The listing builds one solid part. Answer for the finished solid, in the listing's coordinates (mm). Coordinates: 2 decimals unless noted, no trailing zeros. Loops run counter-clockwise (first coordinate to the right, second up) from the corner with the lowest first, then second, coordinate; pieces in that order, holes last. Notation, with made-up numbers: M 67.5,56 L 125.5,56 A16 cw 125.5,72 Z; hole C 37,-38.75 d7. An arc over 180 degrees is marked long. Answer in a Markdown table with one row per item. Add a question column.
from build123d import *

# Parameters (mm, degrees)
SKETCH1_W            = 90
SKETCH1_H            = 55
BOSS_EXTRUDE1_DEPTH  = 16
SKETCH2_W            = 22
SKETCH2_H            = 1.75
SKETCH2_H_2          = 12.5
CUT_EXTRUDE1_DEPTH   = 4
SKETCH3_W            = 20
SKETCH3_H            = 13
CUT_EXTRUDE2_DEPTH   = 20
CHAMFER1_SIZE        = 6
M4_CLEARANCE_HOLE1_D = 4.5
SKETCH7_W            = 27.5
SKETCH7_H            = 8.5
CUT_EXTRUDE3_DEPTH   = 3
SKETCH8_W            = 16.5
SKETCH8_H            = 8.5
CUT_EXTRUDE4_DEPTH   = 12
SKETCH9_R            = 2.25
CUT_EXTRUDE5_DEPTH   = 17
CHAMFER2_SIZE        = 5
SKETCH10_W           = 4
SKETCH10_H           = 22.5
SKETCH10_R           = 2.25
BOSS_EXTRUDE2_DEPTH  = 3


with BuildPart() as part:
    # Sketch1 → Boss-Extrude1 (new body)
    with BuildSketch(Plane(origin=(0, 0, 0), x_dir=(1, 0, 0), z_dir=(0, 1, 0))):
        Rectangle(SKETCH1_W, SKETCH1_H)
    extrude(amount=BOSS_EXTRUDE1_DEPTH)

    # Sketch2 → Cut-Extrude1 (cut)
    with BuildSketch(Plane.ZY.offset(45)):
        with Locations((0, 15.125)):
            Rectangle(SKETCH2_W, SKETCH2_H)
        Polygon((11, 16), (11, 14.25), (13, 14.25), (11.25, 16), align=None)
        Polygon((-11.25, 16), (-13, 14.25), (-11, 14.25), (-11, 16), align=None)
        Polygon((-17.5, 14.25), (-17.5, 1.75), (-13, 1.75), (-11, 1.75), (-11, 14.25), (-13, 14.25), align=None)
        with Locations((0, 8)):
            Rectangle(SKETCH2_W, SKETCH2_H_2)
        Polygon((11, 14.25), (11, 1.75), (13, 1.75), (17.5, 1.75), (17.5, 14.25), (13, 14.25), align=None)
        with Locations((0, 0.875)):
            Rectangle(SKETCH2_W, SKETCH2_H)
        Polygon((13, 1.75), (11, 1.75), (11, 0), (11.25, 0), align=None)
        Polygon((-11, 1.75), (-13, 1.75), (-11.25, 0), (-11, 0), align=None)
    extrude(amount=-CUT_EXTRUDE1_DEPTH, mode=Mode.SUBTRACT)

    # Sketch3 → Cut-Extrude2 (cut)
    with BuildSketch(Plane.ZY.offset(41)):
        with Locations((0, 8)):
            Rectangle(SKETCH3_W, SKETCH3_H)
    extrude(amount=-CUT_EXTRUDE2_DEPTH, mode=Mode.SUBTRACT)

    # Chamfer1
    chamfer1_edges = [part.edges().sort_by_distance(p)[0] for p in [
        (45, 8, 27.5),
        (-45, 8, 27.5),
        (-45, 8, -27.5),
        (45, 8, -27.5),
    ]]
    chamfer(chamfer1_edges, length=CHAMFER1_SIZE)

    # M4 Clearance Hole1 (through all)
    with Locations(Plane(origin=(0, 16, 0), x_dir=(1, 0, 0), z_dir=(0, 1, 0))):
        with Locations((0, 0), (37.5, 20), (-37.5, -20), (-37.5, 20), (37.5, -20)):
            Hole(M4_CLEARANCE_HOLE1_D / 2)

    # Sketch7 → Cut-Extrude3 (cut)
    with BuildSketch(Plane(origin=(45, 0, 0), x_dir=(0, 0, -1), z_dir=(1, 0, 0))):
        with Locations((0, 8)):
            Rectangle(SKETCH7_W, SKETCH7_H)
    extrude(amount=-CUT_EXTRUDE3_DEPTH, mode=Mode.SUBTRACT)

    # Sketch8 → Cut-Extrude4 (cut)
    with BuildSketch(Plane(origin=(42, 0, 0), x_dir=(0, 0, -1), z_dir=(1, 0, 0))):
        with Locations((0, 8)):
            Rectangle(SKETCH8_W, SKETCH8_H)
    extrude(amount=-CUT_EXTRUDE4_DEPTH, mode=Mode.SUBTRACT)

    # Sketch9 → Cut-Extrude5 (cut, through all)
    with BuildSketch(Plane(origin=(0, 16, 0), x_dir=(1, 0, 0), z_dir=(0, 1, 0))):
        Polygon((30, -12.5), (40, -12.5), (40, 12.5), (30, 12.5), (30, 22.5), (-30, 22.5), (-30, 12.5), (-36, 12.5), (-36, -12.5), (-30, -12.5), (-30, -22.5), (30, -22.5), align=None)
        Circle(SKETCH9_R, mode=Mode.SUBTRACT)
    extrude(amount=-CUT_EXTRUDE5_DEPTH, mode=Mode.SUBTRACT)

    # Chamfer2
    chamfer2_edges = [part.edges().sort_by_distance(p)[0] for p in [
        (30, 8, -12.5),
        (30, 8, 12.5),
        (-30, 8, 12.5),
        (-30, 8, -12.5),
    ]]
    chamfer(chamfer2_edges, length=CHAMFER2_SIZE)


with BuildPart() as body_2:
    # Sketch10 → Boss-Extrude2 (new body)
    with BuildSketch(Plane(origin=(0, 16, 0), x_dir=(1, 0, 0), z_dir=(0, 1, 0))):
        with Locations((-43, 0)):
            Rectangle(SKETCH10_W, SKETCH10_H)
        Polygon((39, -27.5), (45, -21.5), (45, 21.5), (39, 27.5), (-39, 27.5), (-45, 21.5), (-45, 11.25), (-41, 11.25), (-41, -11.25), (-45, -11.25), (-45, -21.5), (-39, -27.5), align=None)
        with Locations((37.5, -20)):
            Circle(SKETCH10_R, mode=Mode.SUBTRACT)
        with Locations((-37.5, -20)):
            Circle(SKETCH10_R, mode=Mode.SUBTRACT)
        with Locations((37.5, 20)):
            Circle(SKETCH10_R, mode=Mode.SUBTRACT)
        with Locations((-37.5, 20)):
            Circle(SKETCH10_R, mode=Mode.SUBTRACT)
        Polygon((-36, -12.5), (-36, 12.5), (-35, 12.5), (-30, 17.5), (-30, 22.5), (30, 22.5), (30, 17.5), (35, 12.5), (40, 12.5), (40, -12.5), (35, -12.5), (30, -17.5), (30, -22.5), (-30, -22.5), (-30, -17.5), (-35, -12.5), align=None, mode=Mode.SUBTRACT)
        Polygon((-36, 12.5), (-35, 12.5), (-30, 17.5), (-30, 22.5), (30, 22.5), (30, 17.5), (35, 12.5), (40, 12.5), (40, -12.5), (35, -12.5), (30, -17.5), (30, -22.5), (-30, -22.5), (-30, -17.5), (-35, -12.5), (-36, -12.5), align=None)
    extrude(amount=BOSS_EXTRUDE2_DEPTH)


solid = body_2.part
(1) Straight lines are drawn through the part: line 1 (X direction, y = 18, z = 20); line 2 (Z direction, x = 37.5, y = 17.6); line 3 (X direction, y = 17.7, z = 18.5). For each, find the intervals that lie inside material, in ascending order.
(2) The mould has two halves that part along X. Classify faces 1 (the face through (42, 17.5, 24.5)), 2 (the face through (38.538, 17.479, -18.004)), 3 (the face through (38.538, 17.479, 21.996)), 4 (the face through (1, 17, -27.5)): released by +X, released by -X, zero draft, split by the parting line, or undercut.
(3) A cutting plane is placed at A-A (z = 20). Give the vertices of the cut face in (x, y).
(4) A cutting plane is placed at C-C (y = 17.5). Give the vertices of the cut face in (x, z).
(5) A cutting plane is placed at B-B (x = 37.5). Give the vertices of the cut face in (y, z).
Solved:
| question | item | result |
|---|---|---|
| 1 | line 1 | x = -45 to -39.75, -35.25 to 35.25, 39.75 to 45 |
| 1 | line 2 | z = -27.5 to -22.25, -17.75 to 17.75, 22.25 to 27.5 |
| 1 | line 3 | x = -45 to -39.18, -35.82 to 35.82, 39.18 to 45 |
| 2 | face 1 | released by +X |
| 2 | face 2 | undercut |
| 2 | face 3 | undercut |
| 2 | face 4 | zero draft |
| 3 | outline | M -45,16 L -39.75,16 L -39.75,19 L -45,19 Z; M -35.25,16 L 35.25,16 L 35.25,19 L -35.25,19 Z; M 39.75,16 L 45,16 L 45,19 L 39.75,19 Z |
| 4 | outline | M -45,-21.5 L -39,-27.5 L 39,-27.5 L 45,-21.5 L 45,21.5 L 39,27.5 L -39,27.5 L -45,21.5 Z; hole C -37.5,-20 d4.5; hole C -37.5,20 d4.5; hole C 37.5,-20 d4.5; hole C 37.5,20 d4.5 |
| 5 | outline | M 16,-27.5 L 19,-27.5 L 19,-22.25 L 16,-22.25 Z; M 16,-17.75 L 19,-17.75 L 19,17.75 L 16,17.75 Z; M 16,22.25 L 19,22.25 L 19,27.5 L 16,27.5 Z |
